```python
from build123d import *

# Parameters (mm, degrees)
SKETCH1_W                      = 120
SKETCH1_H                      = 120
BOSS_EXTRUDE1_DEPTH            = 25
M3_CLEARANCE_HOLE1_D           = 3.4
M3_CLEARANCE_HOLE1_CSINK_D     = 3.45
M3_CLEARANCE_HOLE1_CSINK_ANGLE = 100


with BuildPart() as part:
    # Sketch1 → Boss-Extrude1 (new body)
    with BuildSketch(Plane.XY):
        Rectangle(SKETCH1_W, SKETCH1_H)
    extrude(amount=BOSS_EXTRUDE1_DEPTH)

    # M3 Clearance Hole1 (through all)
    with Locations(Plane.XY.offset(25)):
        with Locations((-52.5, 52.5), (52.5, 52.5), (52.5, -52.5), (-52.5, -52.5)):
            CounterSinkHole(M3_CLEARANCE_HOLE1_D / 2, M3_CLEARANCE_HOLE1_CSINK_D / 2, counter_sink_angle=M3_CLEARANCE_HOLE1_CSINK_ANGLE)


solid = part.part
```
Source: CAD feature listing. Evaluate the final solid. Frame: model axes, mm. Round coordinates to 2 decimals unless told otherwise and drop trailing zeros. Loops run counter-clockwise (first coordinate to the right, second up) from the corner with the lowest first, then second, coordinate; pieces in that order, holes last. Notation, with made-up numbers: M 21.5,11.5 L 44.5,11.5 A29 ccw 44.5,42.5 Z; hole C -35,14 d1. An arc over 180 degrees is marked long. Use a Markdown table: item, result. Add a question column.
1. Cut plane A-A, the plane y = 52.5. Output: boundary loops of the cut face in (x, z) (3 decimals), and give its area (3 significant figures).
2. Contact query for a flat-ended pin moving along its axis: pin 1 (2 mm diameter, centred on x = 52.5, y = 52.5, fed in from -Z). Output: stop coordinate, or through.
3. Pull-direction query (X, two-part tool) for faces 1 (the cylindrical face through (54.2, 52.57, 12.31)), 2 (the flat face through (-1, 1, 25)), 3 (the flat face through (60, -1, 12)); classes: +X half, -X half, draft (parallel to the pull), parting line (faces both ways), or undercut.
4. Ray query, line 1 along X through (y, z) = (52.5, 15). Return the intervals inside material, ascending. Write a range as [from, to].
Solution:
| question | item | result |
|---|---|---|
| 1 | outline | M -60,0 L -54.2,0 L -54.2,24.979 L -54.225,25 L -60,25 Z; M -50.8,0 L 50.8,0 L 50.8,24.979 L 50.775,25 L -50.775,25 L -50.8,24.979 Z; M 54.2,0 L 60,0 L 60,25 L 54.225,25 L 54.2,24.979 Z |
| 1 | area | 2,830 mm2 |
| 2 | pin 1 | passes through |
| 3 | face 1 | undercut |
| 3 | face 2 | draft |
| 3 | face 3 | +X half |
| 4 | line 1 | x = [-60, -54.2], [-50.8, 50.8], [54.2, 60] |
